```python
from build123d import *

# Parameters (mm, degrees)
SKETCH1_W           = 279.4
SKETCH1_H           = 57.15
BOSS_EXTRUDE1_DEPTH = 6.35
SKETCH3_W           = 24.892
SKETCH3_H           = 18.542
BOSS_EXTRUDE2_DEPTH = 6.35
SKETCH4_W           = 13.208
SKETCH4_H           = 13.208
CUT_EXTRUDE2_DEPTH  = 148.568371235
SKETCH5_W           = 311.517575851
SKETCH5_H           = 12.7
CUT_EXTRUDE3_DEPTH  = 148.568371235


with BuildPart() as part:
    # Sketch1 → Boss-Extrude1 (new body)
    with BuildSketch(Plane(origin=(0, 0, 0), x_dir=(1, 0, 0), z_dir=(0, 1, 0))):
        Rectangle(SKETCH1_W, SKETCH1_H)
    extrude(amount=BOSS_EXTRUDE1_DEPTH)

    # Sketch3 → Boss-Extrude2 (add)
    with BuildSketch(Plane(origin=(0, 0, 0), x_dir=(1, 0, 0), z_dir=(0, 1, 0))):
        with Locations((-95.25, -37.846)):
            Rectangle(SKETCH3_W, SKETCH3_H)
        with Locations((-57.15, -37.846)):
            Rectangle(SKETCH3_W, SKETCH3_H)
        with Locations((-19.05, -37.846)):
            Rectangle(SKETCH3_W, SKETCH3_H)
        with Locations((19.05, -37.846)):
            Rectangle(SKETCH3_W, SKETCH3_H)
        with Locations((57.15, -37.846)):
            Rectangle(SKETCH3_W, SKETCH3_H)
        with Locations((95.25, -37.846)):
            Rectangle(SKETCH3_W, SKETCH3_H)
    extrude(amount=BOSS_EXTRUDE2_DEPTH)

    # Sketch4 → Cut-Extrude2 (cut, through all)
    with BuildSketch(Plane(origin=(0, 0, 0), x_dir=(1, 0, 0), z_dir=(0, 1, 0))):
        with Locations((-139.7, 9.525)):
            Rectangle(SKETCH4_W, SKETCH4_H)
        with Locations((-139.7, -15.875)):
            Rectangle(SKETCH4_W, SKETCH4_H)
        with Locations((139.7, -15.875)):
            Rectangle(SKETCH4_W, SKETCH4_H)
        with Locations((139.7, 9.525)):
            Rectangle(SKETCH4_W, SKETCH4_H)
    extrude(amount=CUT_EXTRUDE2_DEPTH, mode=Mode.SUBTRACT)

    # Sketch5 → Cut-Extrude3 (cut, through all)
    with BuildSketch(Plane(origin=(0, 6.35, 0), x_dir=(1, 0, 0), z_dir=(0, 1, 0))):
        with Locations((16.058787925, 22.225)):
            Rectangle(SKETCH5_W, SKETCH5_H)
    extrude(amount=-CUT_EXTRUDE3_DEPTH, mode=Mode.SUBTRACT)


solid = part.part
```
Design review of the part built by this model. Coordinates are the model's own, in mm. A direction names the side the tool comes from. Give positions to 0.01 mm unless a question says otherwise; leave off trailing zeros. Write each loop counter-clockwise with the first axis right and the second up, starting at its lowest first coordinate (ties: lowest second). Pieces come first, ordered by that corner, then holes.
(1) Tool access review of faces 1 (the face through (-139.7, 3, 3)), 2 (the face through (-19, 3, 47.117)), 3 (the face through (82.804, 3, 38)), 4 (the face through (133.096, 3, -9)), 5 (the face through (-136, 3, -2.921)): name each direction out of +Z, -Z, +X, -X, +Y, -Y from which nothing blocks a thin tool from reaching the whole face with its end or side.
Checked values:
face 1: +Z, -Z, -X, +Y, -Y
face 2: +Z, +X, -X, +Y, -Y
face 3: +Z, +Y, -Y
face 4: -Z, +X, +Y, -Y
face 5: -Z, -X, +Y, -Y
(2) Clearance check with flat-ended pins moving along their axes: pin 1 Ø1.9 at (x, y) = (0, 4) entering from +Z (3 decimals); pin 2 Ø1.9 at (y, z) = (4.5, 42) entering from +X; pin 3 Ø1.9 at (y, z) = (2, -9.5) entering from -X. State where each tip first meets the part, or that it passes through.
Checked values:
pin 1: stops at z = 28.575
pin 2: stops at x = 107.7
pin 3: stops at x = -133.1
(3) Add section B-B (x = -40). Give the boundary of the cut face in (y, z) (3 decimals).
Checked values:
outline: (0, -15.875) - (6.35, -15.875) - (6.35, 28.575) - (0, 28.575) - close
(4) Add section C-C (z = 20). Give the boundary of the cut face in (x, y).
Checked values:
outline: (-133.1, 0) - (133.1, 0) - (133.1, 6.35) - (-133.1, 6.35) - close
(5) Wall thickness on line 1 along X through (y, z) = (4.25, 29.5); line 2 along X through (y, z) = (5.25, -4); line 3 along Z through (x, y) = (-79, 5.75) (3 decimals): over which ranges is each line inside the solid? List them lowest first.
Checked values:
line 1: x = -107.7 to -82.8, -69.6 to -44.7, -31.5 to -6.6, 6.6 to 31.5, 44.7 to 69.6, 82.8 to 107.7
line 2: x = -133.1 to 133.1
line 3: z = -15.875 to 28.575
(6) Add section A-A (z = 31.5). Give the boundary of the cut face in (x, y).
Checked values:
outline: (-107.7, 0) - (-82.8, 0) - (-82.8, 6.35) - (-107.7, 6.35) - close; (-69.6, 0) - (-44.7, 0) - (-44.7, 6.35) - (-69.6, 6.35) - close; (-31.5, 0) - (-6.6, 0) - (-6.6, 6.35) - (-31.5, 6.35) - close; (6.6, 0) - (31.5, 0) - (31.5, 6.35) - (6.6, 6.35) - close; (44.7, 0) - (69.6, 0) - (69.6, 6.35) - (44.7, 6.35) - close; (82.8, 0) - (107.7, 0) - (107.7, 6.35) - (82.8, 6.35) - close
